The drawing under review shows one solid part. Ordinate dimensions are in mm from its lowest x, y, z. Give positions to 0.01 mm unless a question says otherwise; leave off trailing zeros. Write each loop counter-clockwise with the first axis right and the second up, starting at its lowest first coordinate (ties: lowest second). Pieces come first, ordered by that corner, then holes. Notation, with made-up numbers: (23, 23.25) -> (34, 23.25) arc R21 cw to (34, 38.25) -> close; hole circle Ø6 at (24, 82). An arc over 180 degrees is marked (long way). Answer as a JSON object with one key per item and string values.
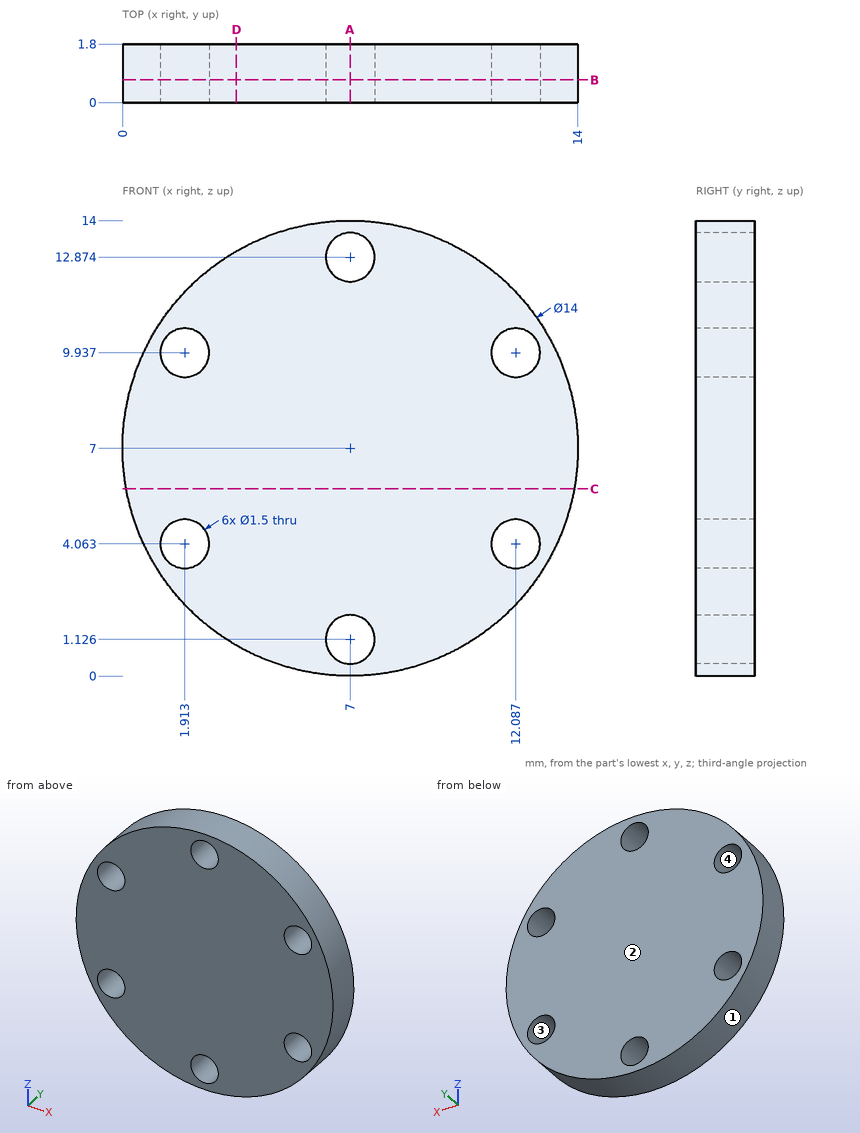
(1) The part is to be moulded in two halves that separate along X. For the marked faces 1, 2, 3 and 4, say which applies: +X half, -X half, draft (parallel to the pull), parting line (faces both ways), or undercut.
Here are the results:
{"face 1": "parting line", "face 2": "draft", "face 3": "undercut", "face 4": "undercut"}
(2) We need section A-A, the plane x = 7. State the section outline as (y, z) points, then the cut area to 3 significant figures.
Here are the results:
{"outline": "(0, 0) -> (1.8, 0) -> (1.8, 0.38) -> (0, 0.38) -> close; (0, 1.88) -> (1.8, 1.88) -> (1.8, 12.12) -> (0, 12.12) -> close; (0, 13.62) -> (1.8, 13.62) -> (1.8, 14) -> (0, 14) -> close", "area": "19.8 mm²"}
(3) Clearance check with flat-ended pins moving along their axes: pin 1 (1.2 mm diameter, centred on x = 1.91, z = 9.94, fed in from -Y); pin 2 (1.7 mm diameter, centred on x = 7, z = 12.87, fed in from +Y). State where each tip first meets the part, or that it passes through.
Here are the results:
{"pin 1": "passes through", "pin 2": "stops at y = 1.8"}
(4) We need section C-C, the plane z = 5.75. State the section outline as (x, y) points.
Here are the results:
{"outline": "(0.11, 0) -> (13.89, 0) -> (13.89, 1.8) -> (0.11, 1.8) -> close"}
(5) We need section D-D, the plane x = 3.5. State the section outline as (y, z) points.
Here are the results:
{"outline": "(0, 0.94) -> (1.8, 0.94) -> (1.8, 13.06) -> (0, 13.06) -> close"}
(6) For line 1 along Z through (x, y) = (6.5, 1.3) (1 decimal); line 2 along X through (y, z) = (1.15, 10.25) (1 decimal); line 3 along Z through (x, y) = (9.25, 1.25), list the stretches that pass through material, from the lowest coordinate up.
Here are the results:
{"line 1": "z = 0 to 0.6, 1.7 to 12.3, 13.4 to 14", "line 2": "x = 0.8 to 1.2, 2.6 to 11.4, 12.8 to 13.2", "line 3": "z = 0.37 to 13.63"}
(7) We need section B-B, the plane y = 0.7. State the section outline as (x, z) points.
Here are the results:
{"outline": "circle Ø14 at (7, 7); hole circle Ø1.5 at (1.91, 4.06); hole circle Ø1.5 at (1.91, 9.94); hole circle Ø1.5 at (7, 1.13); hole circle Ø1.5 at (7, 12.87); hole circle Ø1.5 at (12.09, 4.06); hole circle Ø1.5 at (12.09, 9.94)"}
